Here's the drawing with two shaded views (mm, measured from the low corner). I have some questions. Round coordinates to 2 decimals unless told otherwise and drop trailing zeros. Order: outer loops, then holes, each group sorted by start corner. A loop starts at its lowest first (then second) coordinate and runs counter-clockwise, first axis right, second up.
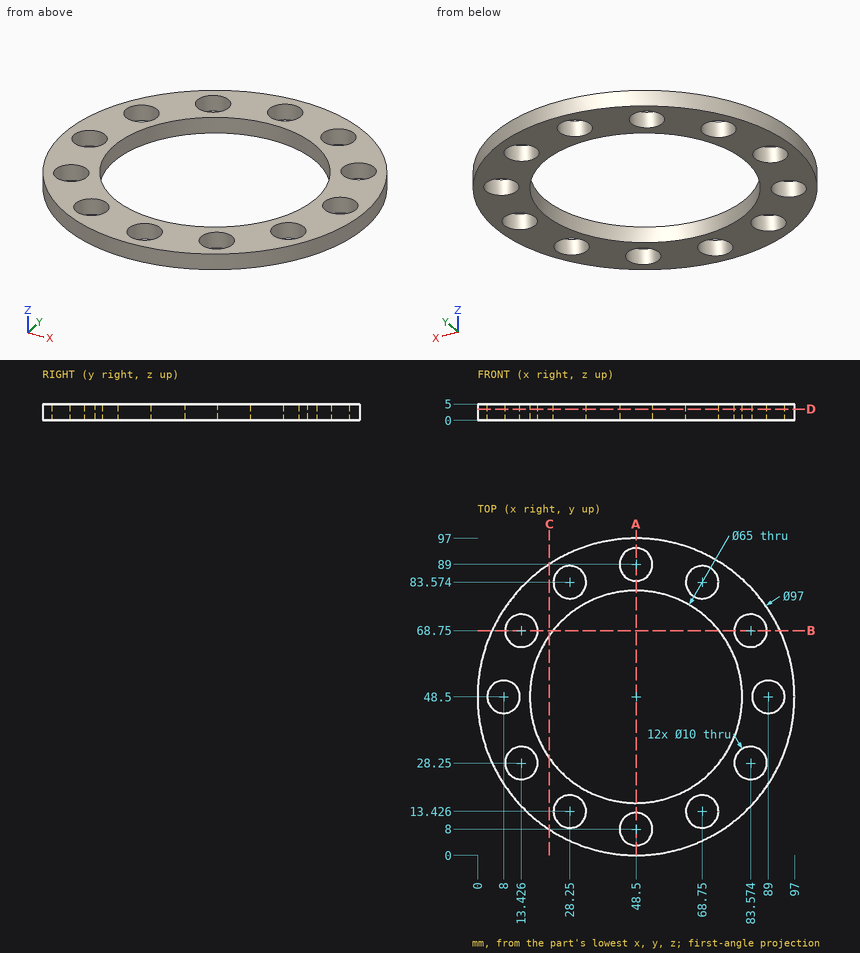
1. If we section it at A-A, the plane x = 48.5: Write out the boundary of the cut face in (y, z).
Evaluation:
outline: (0, 0) - (3, 0) - (3, 5) - (0, 5) - close; (13, 0) - (16, 0) - (16, 5) - (13, 5) - close; (81, 0) - (84, 0) - (84, 5) - (81, 5) - close; (94, 0) - (97, 0) - (97, 5) - (94, 5) - close
2. I need wall thicknesses on probe 1 along X at (y, z) = (11, 2.7); probe 2 along Y at (x, z) = (51.5, 0.6); probe 3 along X at (y, z) = (68, 3.3). Which ranges of each line are inside material? Lowest first, please.
Evaluation:
probe 1: x = 17.74 to 23.88, 32.62 to 44.5, 52.5 to 64.38, 73.12 to 79.26
probe 2: y = 0.09 to 4, 12 to 16.14, 80.86 to 85, 93 to 96.91
probe 3: x = 4.09 to 8.48, 18.37 to 22.5, 74.5 to 78.63, 88.52 to 92.91
3. If we section it at C-C, the plane x = 22: Write out the boundary of the cut face in (y, z), and give its area (3 significant figures).
Evaluation:
outline: (7.88, 0) - (29.69, 0) - (29.69, 5) - (7.88, 5) - close; (67.31, 0) - (89.12, 0) - (89.12, 5) - (67.31, 5) - close
area: 218 mm2
4. I'm going to push flat-ended pins straight in: P1, Ø8, axis at x = 13.43, y = 28.25, coming from the -Z side; P2, Ø1, axis at x = 79, z = 3, coming from the -Y side; P3, Ø1, axis at x = 30.5, z = 4, coming from the -Y side; P4, Ø3, axis at y = 68.5, z = 4.5, coming from the -X side. Where does each tip first touch, or does it pass through?
Evaluation:
P1: passes through
P2: stops at y = 10.39
P3: stops at y = 3.27
P4: stops at x = 3.67
5. If we section it at B-B, the plane y = 68.75: Write out the boundary of the cut face in (x, z).
Evaluation:
outline: (4.43, 0) - (8.43, 0) - (8.43, 5) - (4.43, 5) - close; (18.43, 0) - (23.08, 0) - (23.08, 5) - (18.43, 5) - close; (73.92, 0) - (78.57, 0) - (78.57, 5) - (73.92, 5) - close; (88.57, 0) - (92.57, 0) - (92.57, 5) - (88.57, 5) - close
6. If we section it at D-D, the plane z = 3.4: State how many separate pieces and enclosed holes the cut face has, and give its area (3 significant figures).
Evaluation:
separate pieces: 1
enclosed holes: 13
area: 3,130 mm2
